from build123d import *

# Parameters (mm, degrees)
SKETCH1_R           = 63.5
BOSS_EXTRUDE1_DEPTH = 19.05
SKETCH2_R           = 44.45
CUT_EXTRUDE1_DEPTH  = 92.800885072
SKETCH3_R           = 47.8155
CUT_EXTRUDE2_DEPTH  = 6.35
SKETCH4_R           = 2.5527
CUT_EXTRUDE3_DEPTH  = 92.800885093
SKETCH5_R           = 4.7625
CUT_EXTRUDE4_DEPTH  = 6.35


with BuildPart() as part:
    # Sketch1 → Boss-Extrude1 (new body)
    with BuildSketch(Plane.XY):
        Circle(SKETCH1_R)
    extrude(amount=BOSS_EXTRUDE1_DEPTH)

    # Sketch2 → Cut-Extrude1 (cut, through all)
    with BuildSketch(Plane.XY):
        Circle(SKETCH2_R)
    extrude(amount=CUT_EXTRUDE1_DEPTH, mode=Mode.SUBTRACT)

    # Sketch3 → Cut-Extrude2 (cut)
    with BuildSketch(Plane(origin=(0, 0, 0), x_dir=(0, 0, -1), z_dir=(1, 0, 0))):
        Circle(SKETCH3_R)
    extrude(amount=CUT_EXTRUDE2_DEPTH, mode=Mode.SUBTRACT)

    # Sketch4 → Cut-Extrude3 (cut, through all)
    with BuildSketch(Plane.XY):
        with Locations((63.5, 111.125)):
            Circle(SKETCH4_R)
        with Locations((7.9375, 55.5625)):
            Circle(SKETCH4_R)
        with Locations((63.5, 0)):
            Circle(SKETCH4_R)
        with Locations((119.0625, 55.5625)):
            Circle(SKETCH4_R)
    extrude(amount=CUT_EXTRUDE3_DEPTH, mode=Mode.SUBTRACT)

    # Sketch5 → Cut-Extrude4 (cut)
    with BuildSketch(Plane.XY):
        with Locations((63.5, 111.125)):
            Circle(SKETCH5_R)
        with Locations((7.9375, 55.5625)):
            Circle(SKETCH5_R)
        with Locations((63.5, 0)):
            Circle(SKETCH5_R)
        with Locations((119.0625, 55.5625)):
            Circle(SKETCH5_R)
    extrude(amount=CUT_EXTRUDE4_DEPTH, mode=Mode.SUBTRACT)


solid = part.part
Build history of the part. All positions in model axes, mm. A direction names the side the tool comes from. Coordinates: 2 decimals unless noted, no trailing zeros. Write each loop counter-clockwise with the first axis right and the second up, starting at its lowest first coordinate (ties: lowest second). Pieces come first, ordered by that corner, then holes.
(1) Cut at A-A on y = 0. List the corners of the cut face in (x, z).
(2) Cut at C-C on z = 13. List the corners of the cut face in (x, y).
(3) Mould opens along X. For faces 1 (the cylindrical face through (-63.44, 2.76, 9.39)), 2 (the flat face through (13, 43, 0)), 3 (the cylindrical face through (7.318, 60.284, 3.131)) say: pulls with the +X half, pulls with the -X half, needs draft (parallel to the pull), parting line crosses it, or undercut.
(4) Drill centre lines: line 1 (Y direction, x = 9, z = 15.75); line 2 (Y direction, x = 10, z = 17); line 3 (Y direction, x = 41, z = 4.25). Where is each one in solid material? Low to high.
(5) Pin check, flat tips, straight feed: pin 1 Ø5.5 at (x, y) = (7.94, 55.56) entering from -Z; pin 2 Ø3.5 at (y, z) = (47, 11.5) entering from +X; pin 3 Ø1.5 at (y, z) = (6, 14) entering from -X. Stop position of each tip, or through.
(6) 3-axis set-ups, long thin cutter, end or side, ignore diameter. For faces 4 (the flat face through (6.35, -45, 7)), 5 (the cylindrical face through (58.74, 0.1, 3.13)), 6 (the flat face through (13, 43, 19.05)): which of +Z, -Z, +X, -X, +Y, -Y reach the whole face in a straight line?
(7) Cut at D-D on y = 17.5. List the corners of the cut face in (x, z), and give its area (3 significant figures).
(8) Cut at B-B on x = -10. List the corners of the cut face in (y, z).
Working result:
1. outline: (-63.5, 0) - (-44.45, 0) - (-44.45, 19.05) - (-63.5, 19.05) - close; (44.45, 0) - (58.74, 0) - (58.74, 6.35) - (60.95, 6.35) - (60.95, 19.05) - (44.45, 19.05) - close
2. outline: (63.45, -2.55) arc R2.55 cw to (63.45, 2.55) arc R63.5 ccw (long way) to start; hole (0, -46.01) - (6.35, -46.01) - (6.35, -43.99) arc R44.45 ccw to (6.35, 43.99) - (6.35, 46.01) - (0, 46.01) - (0, 44.45) arc R44.45 ccw to (0, -44.45) - close; hole circle Ø5.11 at (7.94, 55.56)
3. face 1: parting line crosses it
3. face 2: needs draft
3. face 3: undercut
4. line 1: y = -62.86 to -43.53, 43.53 to 53.24, 57.88 to 62.86
4. line 2: y = -62.71 to -43.31, 43.31 to 54.06, 57.07 to 62.71
4. line 3: y = -48.49 to -17.17, 17.17 to 48.49
5. pin 1: stops at z = 6.35
5. pin 2: stops at x = 44.55
5. pin 3: stops at x = -63.28
6. face 4: -Z
6. face 5: -Z, +X
6. face 6: +Z, +X, -X, +Y, -Y
7. outline: (-61.04, 0) - (-40.86, 0) - (-40.86, 19.05) - (-61.04, 19.05) - close; (40.86, 0) - (61.04, 0) - (61.04, 19.05) - (40.86, 19.05) - close
7. area: 769 mm2
8. outline: (-62.71, 0) - (-43.31, 0) - (-43.31, 19.05) - (-62.71, 19.05) - close; (43.31, 0) - (62.71, 0) - (62.71, 19.05) - (43.31, 19.05) - close
